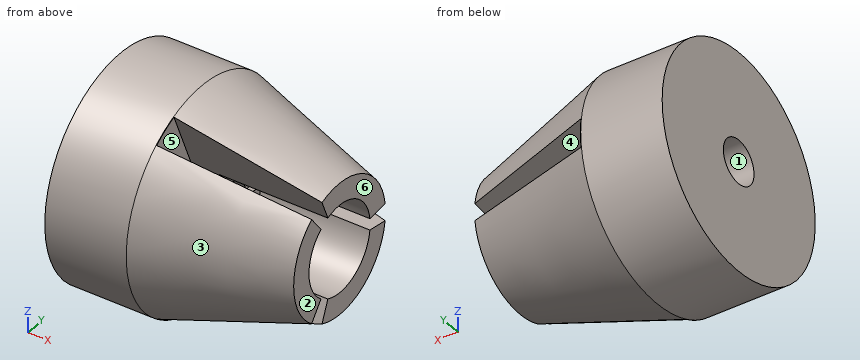
from build123d import *

# Parameters (mm, degrees)
SKETCH3_R          = 2
CUT_EXTRUDE1_DEPTH = 5
SKETCH4_R          = 1
CUT_EXTRUDE2_DEPTH = 5
CUT_EXTRUDE3_DEPTH = 6.25


with BuildPart() as part:
    # Sketch1 → Revolve1 (revolve)
    with BuildSketch(Plane.XY):
        Polygon((0, 0), (0, 5), (3.731538273, 5), (10, 3), (10, 0), align=None)
    revolve(axis=Axis((10, 0, 0), (-1, 0, 0)))

    # Sketch3 → Cut-Extrude1 (cut)
    with BuildSketch(Plane(origin=(10, 0, 0), x_dir=(0, 0, -1), z_dir=(1, 0, 0))):
        with Locations(Location((0, 0, 0), (0, 0, 90))):
            Circle(SKETCH3_R)
    extrude(amount=-CUT_EXTRUDE1_DEPTH, mode=Mode.SUBTRACT)

    # Sketch4 → Cut-Extrude2 (cut)
    with BuildSketch(Plane.ZY):
        with Locations(Location((0, 0, 0), (0, 0, 270))):
            Circle(SKETCH4_R)
    extrude(amount=-CUT_EXTRUDE2_DEPTH, mode=Mode.SUBTRACT)

    # Sketch5 → Cut-Extrude3 (cut)
    with BuildSketch(Plane(origin=(10, 0, 0), x_dir=(0, 0, -1), z_dir=(1, 0, 0))):
        with BuildLine():
            Line((-0.652630961, 4.957224307), (0, 0))
            Line((0, 0), (0.652630961, 4.957224307))
            ThreePointArc((0.652630961, 4.957224307), (0, 5), (-0.652630961, 4.957224307))
        make_face()
        with BuildLine():
            Line((4.619397663, -1.913417162), (0, 0))
            Line((0, 0), (3.966766701, -3.043807145))
            ThreePointArc((3.966766701, -3.043807145), (4.330127019, -2.5), (4.619397663, -1.913417162))
        make_face()
        with BuildLine():
            Line((-3.966766701, -3.043807145), (0, 0))
            Line((0, 0), (-4.619397663, -1.913417162))
            ThreePointArc((-4.619397663, -1.913417162), (-4.330127019, -2.5), (-3.966766701, -3.043807145))
        make_face()
    extrude(amount=-CUT_EXTRUDE3_DEPTH, mode=Mode.SUBTRACT)


solid = part.part
Could you check a few things on this model? Use its own coordinates, in mm. Face numbers are marked on the shaded views. A direction names the side the tool comes from. Give positions to 0.01 mm unless a question says otherwise; leave off trailing zeros. Order: outer loops, then holes, each group sorted by start corner. A loop starts at its lowest first (then second) coordinate and runs counter-clockwise, first axis right, second up. Notation, with made-up numbers: M 43.25,5 L 80.25,5 A35 cw 80.25,42 Z; hole C 30.25,6 d2. An arc over 180 degrees is marked long. One line per question, with ' | ' between items.
1. I want a section at A-A (y = 0). List the corners of the cut face in (x, z) for me.
Results:
outline: M 0,-5 L 3.73,-5 L 10,-3 L 10,-2 L 5,-2 L 5,-1 L 0,-1 Z; M 0,1 L 5,1 L 5,2 L 10,2 L 10,3 L 3.73,5 L 0,5 Z
2. If I drill on line 1 (Z direction, x = 3.4, y = 0); line 2 (X direction, y = 2.5, z = 0.25), over which ranges is the centre line in solid material (lowest first)?
Results:
line 1: -5 to -1, 1 to 5 | line 2: 0 to 3.75
3. We'd pull the mould along Z, two halves only. Please class the marked faces 1, 2 and 3: +Z half, -Z half, draft (parallel to the pull), parting line (faces both ways), or undercut.
Results:
face 1: undercut | face 2: draft | face 3: parting line
4. I'm going to push flat-ended pins straight in: pin 1 (1.1 mm diameter, centred on y = -1, z = 0, fed in from +X); pin 2 (2 mm diameter, centred on x = 3, y = 2.5, fed in from -Z); pin 3 (6 mm diameter, centred on x = 8, y = -2.5, fed in from -Z). Where does each tip first touch, or does it pass through?
Results:
pin 1: x = 5 | pin 2: z = -4.77 | pin 3: z = -4.36
5. I want a section at C-C (x = 2.25). List the corners of the cut face in (y, z) for me.
Results:
outline: C 0,0 d10; hole C 0,0 d2
6. I want a section at D-D (x = 6.5). List the corners of the cut face in (y, z) for me, and give its area (3 significant figures).
Results:
outline: M -2.51,-3.27 L -1.22,-1.59 A2 cw -1.22,1.59 L -2.51,3.27 A4.12 ccw Z; M -1.58,-3.8 A4.12 ccw 4.08,-0.54 L 1.98,-0.26 A2 cw -0.77,-1.85 Z; M -1.58,3.8 L -0.77,1.85 A2 cw 1.98,0.26 L 4.08,0.54 A4.12 ccw Z | area: 35.6 mm²
7. For the marked faces 4, 5 and 6, which set-ups out of +Z, -Z, +X, -X, +Y, -Y let a thin tool reach every point of the face, with its end or its side?
Results:
face 4: +X, +Y | face 5: +X | face 6: +Z, -Z, +X, +Y, -Y
8. I want a section at B-B (x = 4.5). List the corners of the cut face in (y, z) for me, and give its area (3 significant figures).
Results:
outline: M -2.89,-3.77 L -0.61,-0.79 A1 cw -0.61,0.79 L -2.89,3.77 A4.75 ccw Z; M -1.82,-4.39 A4.75 ccw 4.71,-0.62 L 0.99,-0.13 A1 cw -0.38,-0.92 Z; M -1.82,4.39 L -0.38,0.92 A1 cw 0.99,0.13 L 4.71,0.62 A4.75 ccw Z | area: 59.4 mm²
